Verification items for this drawing (mm, ordinates from the low corner). A direction names the side the tool comes from. Coordinates: 2 decimals unless noted, no trailing zeros. Loops run counter-clockwise (first coordinate to the right, second up) from the corner with the lowest first, then second, coordinate; pieces in that order, holes last. Notation, with made-up numbers: M -30,27 L 29,27 A23 ccw 29,43 Z; hole C 16,69 d4. An arc over 180 degrees is marked long. Return JSON: item names as keys, results as strings.
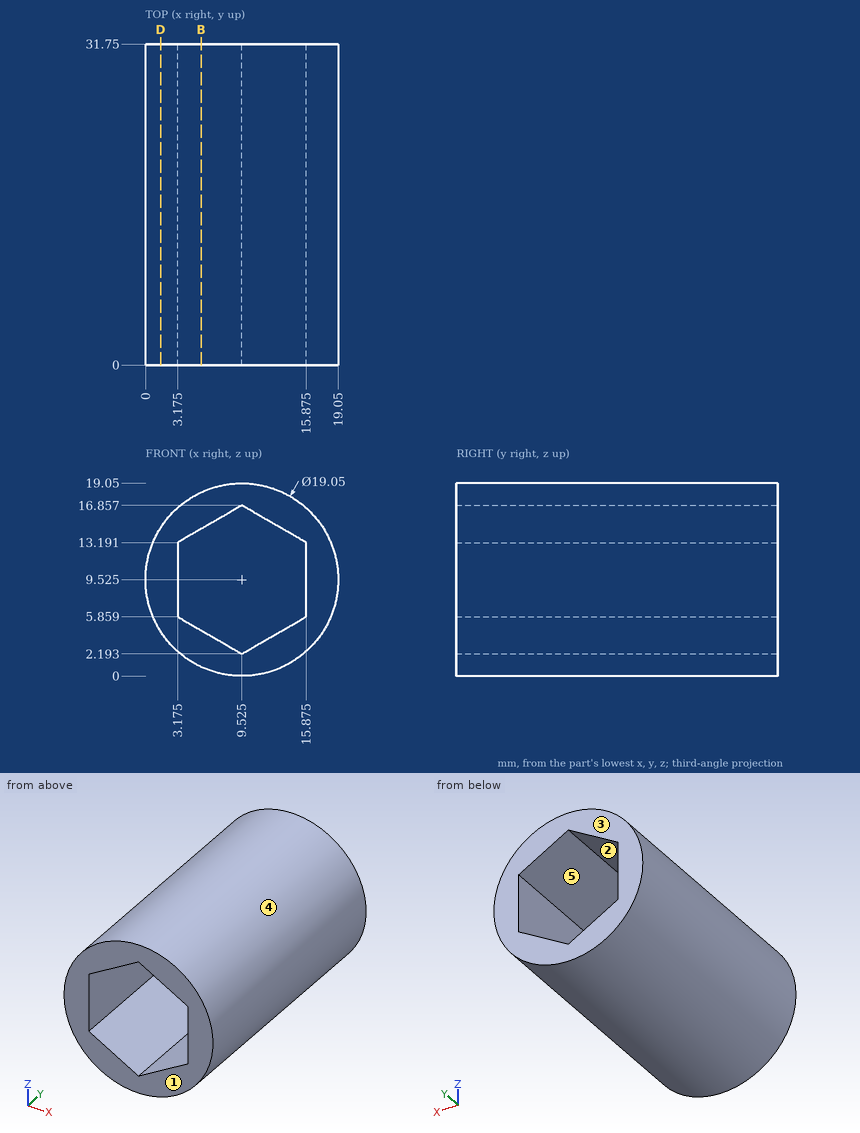
1) Section check D-D on x = 1.5. Record the cut outline in (y, z), then the cut area to 3 significant figures.
Answers:
{"outline": "M 0,4.39 L 31.75,4.39 L 31.75,14.66 L 0,14.66 Z", "area": "326 mm²"}
2) Section check B-B on x = 5.5. Record the cut outline in (y, z), then the cut area to 3 significant figures.
Answers:
{"outline": "M 0,0.89 L 31.75,0.89 L 31.75,4.52 L 0,4.52 Z; M 0,14.53 L 31.75,14.53 L 31.75,18.16 L 0,18.16 Z", "area": "230 mm²"}
3) Set-up check for the marked faces 1 and 2: record each of +Z, -Z, +X, -X, +Y, -Y from which the full face is reachable in a straight line by a thin tool's end or side.
Answers:
{"face 1": "+Z, -Z, +X, -X, -Y", "face 2": "+Y, -Y"}
4) Go/stop test with flat-tipped pins: pin 1 Ø1.5 at (y, z) = (26.5, 7) entering from -X; pin 2 Ø8 at (x, y) = (4.5, 15.5) entering from -Z (1 decimal); pin 3 Ø3 at (x, y) = (2.5, 11) entering from -Z. Record where each tip stops, or that it passes through.
Answers:
{"pin 1": "x = 0.17", "pin 2": "z = 0.1", "pin 3": "z = 1.77"}
5) Draft check along X on the marked faces 3, 4 and 5. Enter one of: +X half, -X half, draft (parallel to the pull), parting line (faces both ways), or undercut.
Answers:
{"face 3": "draft", "face 4": "parting line", "face 5": "undercut"}
6) Scan lines: line 1 along Z through (x, y) = (12.5, 3.5); line 2 along X through (y, z) = (18.5, 5.5) (1 decimal); line 3 along Z through (x, y) = (11.5, 6.5). Record each from-to range of solid material in increasing order. Write a range as [from, to].
Answers:
{"line 1": "[0.48, 3.91], [15.14, 18.57]", "line 2": "[0.9, 3.8], [15.3, 18.2]", "line 3": "[0.21, 3.33], [15.72, 18.84]"}
